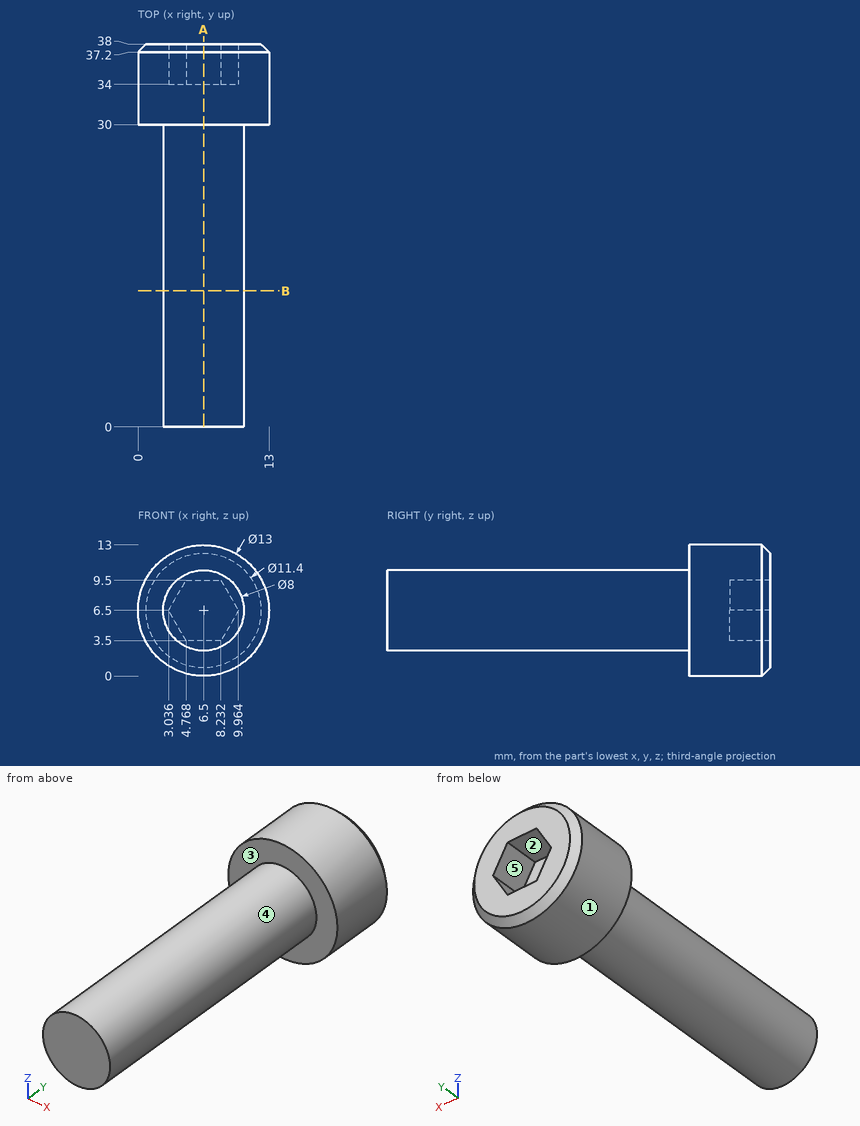
For this review, use the dimensioned drawing (mm, ordinates from the lowest corner) and the shaded views. A direction names the side the tool comes from. Give positions to 0.01 mm unless a question says otherwise; leave off trailing zeros. Write each loop counter-clockwise with the first axis right and the second up, starting at its lowest first coordinate (ties: lowest second). Pieces come first, ordered by that corner, then holes.
(1) Tool access review of the marked faces 1 and 2: name each direction out of +Z, -Z, +X, -X, +Y, -Y from which nothing blocks a thin tool from reaching the whole face with its end or side.
(2) The part is to be moulded in two halves that separate along X. For the marked faces 3, 4 and 5, say which applies: released by +X, released by -X, zero draft, split by the parting line, or undercut.
(3) Consider section B-B, the plane y = 13.5. Give the boundary of the cut face in (x, z).
(4) Consider section A-A, the plane x = 6.5. Give the boundary of the cut face in (y, z), and give its area (3 significant figures).
(5) For P1, Ø4, axis at x = 5.5, y = 10, coming from the -Z side; P2, Ø2, axis at y = 30.5, z = 3.5, coming from the -X side; P3, Ø3, axis at y = 9.5, z = 7, coming from the -X side, all flat-tipped, find the tip position at first contact; note any pin that passes through.
(6) To check wall thickness, follow L1, parallel to Z at x = 6.25, y = 17; L2, parallel to Y at x = 4.75, z = 8.25; L3, parallel to Y at x = 8.25, z = 1.25. State the ranges of each line that lie inside material, in increasing order.
Returned:
1. face 1: +Y, -Y
1. face 2: +Y
2. face 3: zero draft
2. face 4: split by the parting line
2. face 5: undercut
3. outline: circle Ø8 at (6.5, 6.5)
4. outline: (0, 2.5) - (30, 2.5) - (30, 0) - (37.2, 0) - (38, 0.8) - (38, 3.5) - (34, 3.5) - (34, 9.5) - (38, 9.5) - (38, 12.2) - (37.2, 13) - (30, 13) - (30, 10.5) - (0, 10.5) - close
4. area: 319 mm2
5. P1: stops at z = 2.5
5. P2: stops at x = 0.32
5. P3: stops at x = 2.5
6. L1: z = 2.51 to 10.49
6. L2: y = 0 to 34
6. L3: y = 30 to 38
